Can you work these out from the drawing? Everything is in mm from the part's minimum corner. Coordinates: 2 decimals unless noted, no trailing zeros. Write each loop counter-clockwise with the first axis right and the second up, starting at its lowest first coordinate (ties: lowest second). Pieces come first, ordered by that corner, then holes. Notation, with made-up numbers: M 68,84 L 99,84 A10 cw 99,95 Z; hole C 11.5,3 d10. An arc over 180 degrees is marked long. Answer as a JSON object with one key per item and string values. Group by question number.
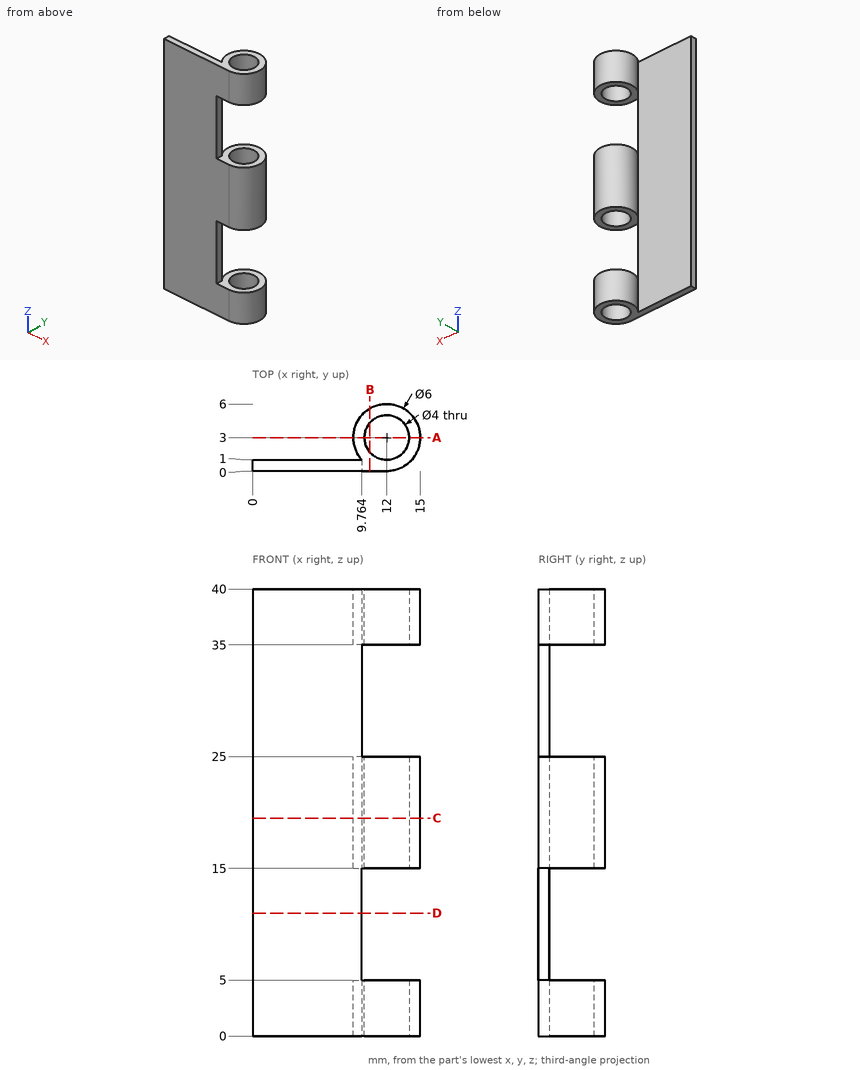
Q1. If we section it at D-D on z = 11: List the corners of the cut face in (x, y) for me.
Q2. If we section it at A-A on y = 3: List the corners of the cut face in (x, z) for me.
Q3. If we section it at C-C on z = 19.5: List the corners of the cut face in (x, y) for me.
Q4. If we section it at B-B on x = 10.5: List the corners of the cut face in (y, z) for me.
Q5. Will these pins go through, and if not, where does the flat tip stop? pin 1 (1.1 mm diameter, centred on y = 0.5, z = 8, fed in from +X); pin 2 (2 mm diameter, centred on x = 4.5, z = 33.5, fed in from +Y); pin 3 (4 mm diameter, centred on x = 7.5, z = 15.5, fed in from +Y).
Q6. Please list where these lines run through material, in increasing order: L1, parallel to X at y = 3, z = 4; L2, parallel to Y at x = 12, z = 2; L3, parallel to Y at x = 3, z = 15.5.
Reply:
{
 "1": {"outline": "M 0,0 L 9.76,0 L 9.76,1 L 0,1 Z"},
 "2": {"outline": "M 9,0 L 10,0 L 10,5 L 9,5 Z; M 9,15 L 10,15 L 10,25 L 9,25 Z; M 9,35 L 10,35 L 10,40 L 9,40 Z; M 14,0 L 15,0 L 15,5 L 14,5 Z; M 14,15 L 15,15 L 15,25 L 14,25 Z; M 14,35 L 15,35 L 15,40 L 14,40 Z"},
 "3": {"outline": "M 0,0 L 12,0 A3 ccw long 9.76,1 L 0,1 Z; hole C 12,3 d4"},
 "4": {"outline": "M 0,0 L 1.68,0 L 1.68,5 L 0,5 Z; M 0,15 L 1.68,15 L 1.68,25 L 0,25 Z; M 0,35 L 1.68,35 L 1.68,40 L 0,40 Z; M 4.32,0 L 5.6,0 L 5.6,5 L 4.32,5 Z; M 4.32,15 L 5.6,15 L 5.6,25 L 4.32,25 Z; M 4.32,35 L 5.6,35 L 5.6,40 L 4.32,40 Z"},
 "5": {"pin 1": "x = 9.76", "pin 2": "y = 1", "pin 3": "y = 4.66"},
 "6": {"L1": "9 to 10, 14 to 15", "L2": "0 to 1, 5 to 6", "L3": "0 to 1"}
}
